from build123d import *

# Parameters (mm, degrees)
F0_W      = 152.4
F0_H      = 114.3
F1_DEPTH  = 152.4
F2_W      = 19.05
F2_H      = 78.74
F3_DEPTH  = 152.401
F4_DEPTH  = 152.401
F5_W      = 73.66
F5_H      = 50.8
F5_H_2    = 25.4
F6_DEPTH  = 114.301
F7_W      = 73.66
F7_H      = 12.7
F8_DEPTH  = 114.301
F9_DEPTH  = 25.4
F10_W     = 73.456201
F10_H     = 38.1
F11_DEPTH = 50.8


with BuildPart() as f1:
    # F0 (on Front) → F1 (new body)
    with BuildSketch(Plane.XZ):
        Rectangle(F0_W, F0_H)
    extrude(amount=F1_DEPTH)

    # F2 (on face) → F3 (cut, through all)
    with BuildSketch(Plane.XZ.offset(152.4)):
        with Locations((-66.675, 0)):
            Rectangle(F2_W, F2_H)
    extrude(amount=-F3_DEPTH, mode=Mode.SUBTRACT)

    # F2 (on face) → F4 (cut, through all)
    with BuildSketch(Plane.XZ.offset(152.4)):
        with Locations((66.675, 0)):
            Rectangle(F2_W, F2_H)
    extrude(amount=-F4_DEPTH, mode=Mode.SUBTRACT)

    # F5 (on face) → F6 (cut, through all)
    with BuildSketch(Plane.XY.offset(57.15)):
        with Locations((0.203799, -127)):
            Rectangle(F5_W, F5_H)
        with Locations((0.203799, -12.7)):
            Rectangle(F5_W, F5_H_2)
    extrude(amount=-F6_DEPTH, mode=Mode.SUBTRACT)

    # F7 (on face) → F8 (cut, through all)
    with BuildSketch(Plane.XY.offset(57.15)):
        with Locations((0, -57.15)):
            Rectangle(F7_W, F7_H)
    extrude(amount=-F8_DEPTH, mode=Mode.SUBTRACT)

    # F7 (on face) → F9 (cut)
    with BuildSketch(Plane.XY.offset(57.15)):
        Polygon((-36.83, -63.5), (-36.83, -101.6), (-36.626201, -101.6), (36.83, -101.6), (36.83, -63.5), align=None)
    extrude(amount=-F9_DEPTH, mode=Mode.SUBTRACT)

    # F10 (on face) → F11 (cut)
    with BuildSketch(Plane(origin=(0, 0, -57.15), x_dir=(1, 0, 0), z_dir=(0, 0, -1))):
        with Locations((0.101899, 82.55)):
            Rectangle(F10_W, F10_H)
    extrude(amount=-F11_DEPTH, mode=Mode.SUBTRACT)


solid = f1.part
Can you work these out from the model? Positions are in its coordinate system, mm. A direction names the side the tool comes from. Give positions to 0.01 mm unless a question says otherwise; leave off trailing zeros. Write each loop counter-clockwise with the first axis right and the second up, starting at its lowest first coordinate (ties: lowest second). Pieces come first, ordered by that corner, then holes. Notation, with made-up numbers: (87.5, -25.5) -> (138.5, -25.5) arc R19 ccw to (138.5, -8.5) -> close; hole circle Ø9 at (31, 25). An arc over 180 degrees is marked (long way). Answer as a JSON object with one key per item and string values. Group by question number.
Item 1: For faces 5 (the face through (0, -25.4, 1)), 6 (the face through (-36.83, -60, 26)), 7 (the face through (3, -101.6, 13)), 8 (the face through (57.15, -77, -1)), 9 (the face through (-67, -77, 39.37)), which set-ups out of +Z, -Z, +X, -X, +Y, -Y let a thin tool reach every point of the face, with its end or its side?
Item 2: We'd pull the mould along X, two halves only. Please class faces 1 (the face through (-76.2, -75, 48)), 2 (the face through (-1, -50.8, 1)), 3 (the face through (-36.626, -13, 1)), 4 (the face through (-1, -41, 57.15)): +X half, -X half, draft (parallel to the pull), parting line (faces both ways), or undercut.
Item 3: Suppose I cut it at D-D (z = 47). Please give me the cut outline in (x, y), plus the area to 3 significant figures.
Item 4: Please list where these lines run through material, in increasing order: line 1 (X direction, y = -121, z = 28.5); line 2 (X direction, y = -86, z = -21); line 3 (Z direction, x = -61.5, y = -116). Write a range as [from, to].
Item 5: Suppose I cut it at A-A (y = -142). Please give me the cut outline in (x, z).
Item 6: Suppose I cut it at C-C (x = -28.5). Please give me the cut outline in (y, z), plus the area to 3 significant figures.
Item 7: I'm going to push flat-ended pins straight in: P1, Ø12, axis at x = -23, z = 36, coming from the +Y side; P2, Ø5, axis at x = 29, y = -70, coming from the -Z side; P3, Ø12, axis at x = 7, z = -25.5, coming from the -Y side. Where does each tip first touch, or does it pass through?
Item 8: Suppose I cut it at B-B (z = 10.5). Please give me the cut outline in (x, y).
Findings:
{
 "1": {"face 5": "+Z, -Z, +Y", "face 6": "+Z", "face 7": "+Z, -Z, -Y", "face 8": "+X, +Y, -Y", "face 9": "-X, +Y, -Y"},
 "2": {"face 1": "-X half", "face 2": "undercut", "face 3": "undercut", "face 4": "draft"},
 "3": {"outline": "(-76.2, -152.4) -> (-36.63, -152.4) -> (-36.63, -101.6) -> (-36.83, -101.6) -> (-36.83, -50.8) -> (36.83, -50.8) -> (36.83, -101.6) -> (37.03, -101.6) -> (37.03, -152.4) -> (76.2, -152.4) -> (76.2, 0) -> (37.03, 0) -> (37.03, -25.4) -> (-36.63, -25.4) -> (-36.63, 0) -> (-76.2, 0) -> close", "area": "13,900 mm²"},
 "4": {"line 1": "x = [-57.15, -36.63], [37.03, 57.15]", "line 2": "x = [-57.15, -36.63], [36.83, 57.15]", "line 3": "z = [-57.15, -39.37], [39.37, 57.15]"},
 "5": {"outline": "(-76.2, -57.15) -> (-36.63, -57.15) -> (-36.63, 57.15) -> (-76.2, 57.15) -> (-76.2, 39.37) -> (-57.15, 39.37) -> (-57.15, -39.37) -> (-76.2, -39.37) -> close; (37.03, -57.15) -> (76.2, -57.15) -> (76.2, -39.37) -> (57.15, -39.37) -> (57.15, 39.37) -> (76.2, 39.37) -> (76.2, 57.15) -> (37.03, 57.15) -> close"},
 "6": {"outline": "(-101.6, -6.35) -> (-63.5, -6.35) -> (-63.5, 31.75) -> (-101.6, 31.75) -> close; (-50.8, -57.15) -> (-25.4, -57.15) -> (-25.4, 57.15) -> (-50.8, 57.15) -> close", "area": "4,350 mm²"},
 "7": {"P1": "stops at y = -25.4", "P2": "stops at z = -6.35", "P3": "stops at y = -50.8"},
 "8": {"outline": "(-57.15, -152.4) -> (-36.63, -152.4) -> (-36.63, -101.6) -> (37.03, -101.6) -> (37.03, -152.4) -> (57.15, -152.4) -> (57.15, 0) -> (37.03, 0) -> (37.03, -25.4) -> (-36.63, -25.4) -> (-36.63, 0) -> (-57.15, 0) -> close; hole (-36.83, -63.5) -> (36.83, -63.5) -> (36.83, -50.8) -> (-36.83, -50.8) -> close"}
}
